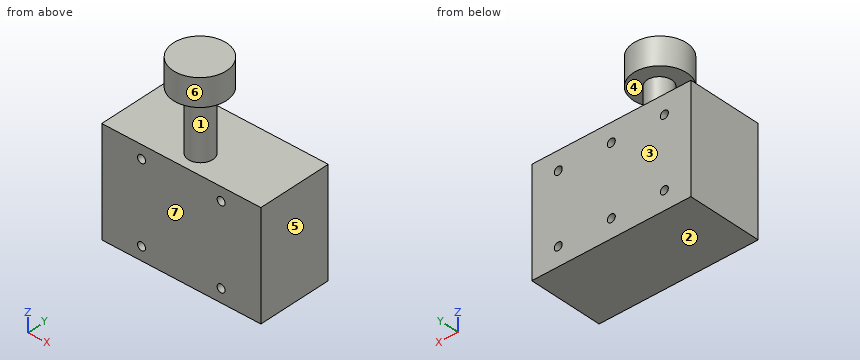
Autodesk Inventor part; units mm, degrees
ref_plane "YZ Plane" through (0, 0, 0) normal (1, 0, 0) x (0, 1, 0)
ref_plane "XZ Plane" through (0, 0, 0) normal (0, 1, 0) x (-1, 0, 0)
ref_plane "XY Plane" through (0, 0, 0) normal (0, 0, 1) x (1, 0, 0)
sketch "Sketch1" plane through (0, 0, 0) normal (0, 1, 0) x (-1, 0, 0)
  line L0 (0, 0) -> (60, 0)
  line L1 (60, 0) -> (60, -40)
  line L2 (60, -40) -> (0, -40)
  line L3 (0, -40) -> (0, 0)
  dimension "d0" = 60
  dimension "d1" = 40
extrude "Extrusion1" add sketch "Sketch1" along normal blind 28
sketch "Sketch2" plane through (-60, 0, 0) normal (0, 0, 1) x (1, 0, 0)
  circle A0 centre (30, 8) radius 4.6
  line L0 (60, 0) -> (60, 28)
  line L1 (60, 0) -> (0, 0)
  dimension "d4" = 9.2
  dimension "d5" = 30
  dimension "d6" = 8
extrude "Extrusion2" add sketch "Sketch2" along normal blind 23
sketch "Sketch3" plane through (-30, 8, 23) normal (0, 0, 1) x (1, 0, 0)
  circle A0 centre (0, 0) radius 4.6
  circle A1 centre (0, -0.2633) radius 10
  point P0 (30, -8)
  dimension "d9" = 20
extrude "Extrusion3" add sketch "Sketch3" along normal blind 10.25 contours A0 | A1
sketch "Sketch4" plane through (0, 0, 0) normal (0, -1, 0) x (1, 0, 0)
  line L0 (0, 0) -> (-60, 0)
  line L1 (-60, 0) -> (-60, -40)
  line L2 (-60, -40) -> (0, -40)
  line L3 (0, -40) -> (0, 0)
  line L4 (-45, -35) -> (-15, -35)
  line L5 (-15, -35) -> (-15, -5)
  line L6 (-15, -5) -> (-45, -5)
  line L7 (-45, -5) -> (-45, -35)
  line L8 (-45, -35) -> (-15, -5) construction
  line L9 (-15, -35) -> (-45, -5) construction
  point P0 (-30, -20)
  dimension "d12" = 30
  dimension "d13" = 30
hole "Hole1" at (-15, 0, -5) at (-15, 0, -35) at (-45, 0, -35) at (-45, 0, -5) direction (0, 1, 0) diameter 3 depth 8 tip angle 118
sketch "Sketch5" plane through (0, 28, 0) normal (0, 1, 0) x (1, 0, 0)
  line L0 (-60, 0) -> (0, 0)
  line L1 (0, 0) -> (0, 40)
  line L2 (0, 40) -> (-60, 40)
  line L3 (-60, 40) -> (-60, 0)
  line L4 (-10, 7) -> (-50, 7)
  line L5 (-50, 7) -> (-50, 33)
  line L6 (-50, 33) -> (-10, 33)
  line L7 (-10, 33) -> (-10, 7)
  line L8 (-10, 7) -> (-50, 33) construction
  line L9 (-50, 7) -> (-10, 33) construction
  point P0 (-30, 20)
  point P1 (-30, 7)
  point P2 (-30, 33)
  dimension "d21" = 40
  dimension "d22" = 26
hole "Hole2" at (-30, 28, -7) at (-30, 28, -33) at (-50, 28, -7) at (-50, 28, -33) at (-10, 28, -33) at (-10, 28, -7) direction (0, -1, 0) diameter 3 depth 8 tip angle 118
properties part number "00_Z-stage"
The model under review builds one solid part; all positions refer to its coordinate system, in mm. Face numbers are marked on the shaded views. A direction names the side the tool comes from. Give positions to 0.01 mm unless a question says otherwise; leave off trailing zeros. Loops run counter-clockwise (first coordinate to the right, second up) from the corner with the lowest first, then second, coordinate; pieces in that order, holes last. Notation, with made-up numbers: (-11, 35) -> (33, 35) arc R19 cw to (33, 53) -> close; hole circle Ø7 at (70, 55). An arc over 180 degrees is marked (long way). Answer as a JSON object with one key per item and string values. Group by question number.
Q1. Take a section at A-A (y = 22). Write out the cut boundary in (x, z).
Q2. Draft analysis for pull direction Z (two halves, no side actions). For the marked faces 1, 2, 3 and 4, state which applies: pulls with the +Z half, pulls with the -Z half, needs draft (parallel to the pull), parting line crosses it, or undercut.
Q3. Insertion check: pin 1 (2.5 mm diameter, centred on x = -10, z = -33, fed in from -Y); pin 2 (2.5 mm diameter, centred on x = -15, z = -35, fed in from -Y); pin 3 (6 mm diameter, centred on y = 5, z = 4, fed in from +X); pin 4 (10 mm diameter, centred on x = -40.5, z = 14, fed in from -Y). Each pin has a flat end and moves straight along its axis. Give the tip position at first contact, or say it passes through.
Q4. Tool access review of the marked faces 5, 6 and 7: name each direction out of +Z, -Z, +X, -X, +Y, -Y from which nothing blocks a thin tool from reaching the whole face with its end or side.
Q5. Wall thickness on line 1 along Z through (x, y) = (-45, 6); line 2 along Z through (x, y) = (-50, 23.5); line 3 along X through (y, z) = (23, -7): over which ranges is each line inside the solid? List them lowest first.
Q6. Take a section at B-B (z = 16.5). Write out the cut boundary in (x, y), plus the area to 3 significant figures.
Q7. Take a section at D-D (y = 10.5). Write out the cut boundary in (x, z), plus the area to 3 significant figures.
Q8. Take a section at C-C (x = -27). Write out the cut boundary in (y, z), plus the area to 3 significant figures.
Answer below:
{
 "1": {"outline": "(-60, -40) -> (0, -40) -> (0, 0) -> (-60, 0) -> close; hole circle Ø3 at (-50, -33); hole circle Ø3 at (-50, -7); hole circle Ø3 at (-30, -33); hole circle Ø3 at (-30, -7); hole circle Ø3 at (-10, -33); hole circle Ø3 at (-10, -7)"},
 "2": {"face 1": "undercut", "face 2": "pulls with the -Z half", "face 3": "needs draft", "face 4": "undercut"},
 "3": {"pin 1": "stops at y = 0", "pin 2": "stops at y = 8.15", "pin 3": "stops at x = -25.4", "pin 4": "passes through"},
 "4": {"face 5": "+Z, -Z, +X, +Y, -Y", "face 6": "+Z", "face 7": "-Z, +X, -X, -Y"},
 "5": {"line 1": "z = -40 to -36.5, -33.5 to -6.5, -3.5 to 0", "line 2": "z = -40 to -34.5, -31.5 to -8.5, -5.5 to 0", "line 3": "x = -60 to -51.5, -48.5 to -31.5, -28.5 to -11.5, -8.5 to 0"},
 "6": {"outline": "circle Ø9.2 at (-30, 8)", "area": "66.5 mm2"},
 "7": {"outline": "(-60, -40) -> (0, -40) -> (0, 0) -> (-26.14, 0) -> (-26.14, 23) -> (-20.39, 23) -> (-20.39, 33.25) -> (-39.61, 33.25) -> (-39.61, 23) -> (-33.86, 23) -> (-33.86, 0) -> (-60, 0) -> close", "area": "2,770 mm2"},
 "8": {"outline": "(-1.8, 23) -> (4.51, 23) -> (4.51, 0) -> (0, 0) -> (0, -40) -> (28, -40) -> (28, 0) -> (11.49, 0) -> (11.49, 23) -> (17.28, 23) -> (17.28, 33.25) -> (-1.8, 33.25) -> close", "area": "1,480 mm2"}
}
